from build123d import *

# Parameters (mm, degrees)
SKETCH_1_R          = 2.7
SKETCH_1_R_2        = 1.5
EXTRUDE_1_DEPTH     = 40
CUT_EXTRUDE_START   = -40
CUT_EXTRUDE_1_DEPTH = 40


with BuildPart() as part:
    # 草图1 → 凸台-拉伸1 (new body)
    with BuildSketch(Plane(origin=(0, 0, 0), x_dir=(1, 0, 0), z_dir=(0, 1, 0))):
        with Locations(Location((0, 0, 0), (0, 0, 270))):
            Circle(SKETCH_1_R)
        with Locations(Location((0, 0, 0), (0, 0, 270))):
            Circle(SKETCH_1_R_2, mode=Mode.SUBTRACT)
    extrude(amount=EXTRUDE_1_DEPTH)

    # 草图2 → 切除-拉伸1 (cut)
    with BuildSketch(Plane(origin=(0, 40, 0), x_dir=(1, 0, 0), z_dir=(0, 1, 0)).offset(CUT_EXTRUDE_START)):
        with BuildLine():
            Line((-2.33826859, 1.35), (0, 2.7))
            ThreePointArc((0, 2.7), (-1.35, 2.33826859), (-2.33826859, 1.35))
        make_face()
        with BuildLine():
            Line((-2.33826859, -1.35), (-2.33826859, 1.35))
            ThreePointArc((-2.33826859, 1.35), (-2.7, 0), (-2.33826859, -1.35))
        make_face()
        with BuildLine():
            Line((0, -2.7), (-2.33826859, -1.35))
            ThreePointArc((-2.33826859, -1.35), (-1.35, -2.33826859), (0, -2.7))
        make_face()
        with BuildLine():
            ThreePointArc((0, -2.7), (1.35, -2.33826859), (2.33826859, -1.35))
            Line((2.33826859, -1.35), (0, -2.7))
        make_face()
        with BuildLine():
            ThreePointArc((2.7, 0), (2.607999731, 0.698811422), (2.33826859, 1.35))
            Line((2.33826859, 1.35), (2.33826859, -1.35))
            ThreePointArc((2.33826859, -1.35), (2.607999731, -0.698811422), (2.7, 0))
        make_face()
        with BuildLine():
            ThreePointArc((2.33826859, 1.35), (1.35, 2.33826859), (0, 2.7))
            Line((0, 2.7), (2.33826859, 1.35))
        make_face()
    extrude(amount=CUT_EXTRUDE_1_DEPTH, mode=Mode.SUBTRACT)


solid = part.part
Can you work these out from the model? Positions are in its coordinate system, mm. Give positions to 0.01 mm unless a question says otherwise; leave off trailing zeros. Write each loop counter-clockwise with the first axis right and the second up, starting at its lowest first coordinate (ties: lowest second). Pieces come first, ordered by that corner, then holes. Notation, with made-up numbers: M 76,11.5 L 129,11.5 A11 cw 129,15.5 Z; hole C -36,76.5 d4. An arc over 180 degrees is marked long. Answer in a Markdown table with one row per item. Add a question column.
Item 1: For pin 1 Ø1 at (x, y) = (-1.5, 27) entering from +Z; pin 2 Ø1.5 at (x, y) = (0.5, 33) entering from -Z, each with a flat end and sliding along its axis, tell me the tip position at first contact or that it passes through.
Item 2: Please list where these lines run through material, in increasing order: L1, parallel to X at y = 24.5, z = 0; L2, parallel to Z at x = 0.8, y = 12; L3, parallel to X at y = 10, z = -0.5.
Item 3: We'd pull the mould along X, two halves only. Please class faces 1 (the cylindrical face through (0.45, 19.72, 1.43)), 2 (the flat face through (2.338, 20, 0)), 3 (the flat face through (2, 40, 0)): released by +X, released by -X, zero draft, split by the parting line, or undercut.
Item 4: Imagine slicing it at B-B, the plane y = 26. Write out the boundary of the cut face in (x, z), plus the area to 3 significant figures.
Item 5: Imagine slicing it at A-A, the plane z = 0. Write out the boundary of the cut face in (x, y), plus the area to 3 significant figures.
Item 6: Imagine slicing it at C-C, the plane z = 2.35. Write out the boundary of the cut face in (x, y), plus the area to 3 significant figures.
Item 7: Imagine slicing it at D-D, the plane x = -1.95. Write out the boundary of the cut face in (y, z).
Evaluation:
| question | item | result |
|---|---|---|
| 1 | pin 1 | stops at z = 2.12 |
| 1 | pin 2 | stops at z = -2.7 |
| 2 | L1 | x = -2.34 to -1.5, 1.5 to 2.34 |
| 2 | L2 | z = -2.24 to -1.27, 1.27 to 2.24 |
| 2 | L3 | x = -2.34 to -1.41, 1.41 to 2.34 |
| 3 | face 1 | undercut |
| 3 | face 2 | released by +X |
| 3 | face 3 | zero draft |
| 4 | outline | M -2.34,-1.35 L 0,-2.7 L 2.34,-1.35 L 2.34,1.35 L 0,2.7 L -2.34,1.35 Z; hole C 0,0 d3 |
| 4 | area | 11.9 mm² |
| 5 | outline | M -2.34,0 L -1.5,0 L -1.5,40 L -2.34,40 Z; M 1.5,0 L 2.34,0 L 2.34,40 L 1.5,40 Z |
| 5 | area | 67.1 mm² |
| 6 | outline | M -0.61,0 L 0.61,0 L 0.61,40 L -0.61,40 Z |
| 6 | area | 48.5 mm² |
| 7 | outline | M 0,-1.57 L 40,-1.57 L 40,1.57 L 0,1.57 Z |
